Geometry check sheet. Reference: the model listing, model coordinates, mm. Face numbers are marked on the shaded views. A direction names the side the tool comes from. Give positions to 0.01 mm unless a question says otherwise; leave off trailing zeros. Order: outer loops, then holes, each group sorted by start corner. A loop starts at its lowest first (then second) coordinate and runs counter-clockwise, first axis right, second up. Notation, with made-up numbers: M 61,79 L 114,79 A29 cw 114,103 Z; hole C 24.25,65 d4. An arc over 180 degrees is marked long. Answer as CSV lines item,"result". Start each with the question number.
Q1. Section check A-A, the plane x = 60.4. Record the boundary of the cut face in (y, z).
Q2. Thickness scan on line 1 (Z direction, x = 37, y = 13.6); line 2 (Z direction, x = 20.5, y = 13.35); line 3 (X direction, y = 13.5, z = -188). Record the ranges inside material, lowest first.
Q3. Section check D-D, the plane z = -173. Record the boundary of the cut face in (x, y).
Q4. Go/stop test with flat-tipped pins: pin 1 (0.8 mm diameter, centred on y = 14, z = -108.5, fed in from +X); pin 2 (22 mm diameter, centred on x = 62, z = -86, fed in from -Y); pin 3 (1.3 mm diameter, centred on y = 14, z = -50.5, fed in from +X). Record where each tip stops, or that it passes through.
Q5. Set-up check for the marked faces 1 and 2: record each of +Z, -Z, +X, -X, +Y, -Y from which the full face is reachable in a straight line by a thin tool's end or side.
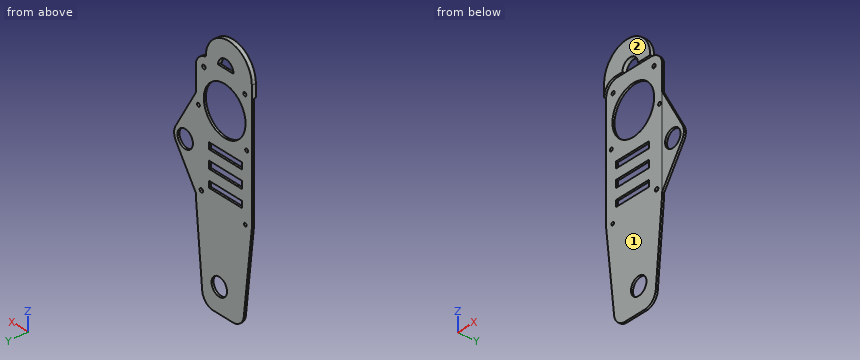
```python
from build123d import *

# Parameters (mm, degrees)
SKETCH1_R           = 2.875
SKETCH1_R_2         = 7
BOSS_EXTRUDE1_DEPTH = 24.5875
SKETCH4_W           = 66.272407177
SKETCH4_H           = 27.800260981
CUT_EXTRUDE2_DEPTH  = 20
FILLET3_R           = 10
FILLET4_R           = 10
BOSS_EXTRUDE3_START = -1.5875
BOSS_EXTRUDE3_DEPTH = 1.5875
SKETCH7_R           = 7
CUT_EXTRUDE3_DEPTH  = 1.5875
CUT_EXTRUDE4_START  = -10
SKETCH8_R           = 3
SKETCH8_R_2         = 18.9
SKETCH8_R_3         = 2.875
SKETCH8_R_4         = 7
CUT_EXTRUDE4_DEPTH  = 10
SKETCH9_W           = 229.1070397
SKETCH9_H           = 361.266964835
SKETCH9_R           = 1.388229101
SKETCH9_R_2         = 1.483383261
SKETCH9_R_3         = 1.314910669
SKETCH9_R_4         = 1.248623853
SKETCH9_R_5         = 1.255629307
SKETCH9_R_6         = 1.53911217
CUT_EXTRUDE5_DEPTH  = 13
SKETCH10_W          = 29.988446547
SKETCH10_H          = 5
SKETCH10_H_2        = 5.75
CUT_EXTRUDE6_DEPTH  = 22
SKETCH11_R          = 5.236653548
CUT_EXTRUDE7_DEPTH  = 10
BOSS_EXTRUDE4_START = -1.59
BOSS_EXTRUDE4_DEPTH = 1.59
SKETCH13_R          = 7
CUT_EXTRUDE8_DEPTH  = 41
SKETCH14_W          = 61.491848917
SKETCH14_H          = 35.587491391
CUT_EXTRUDE9_DEPTH  = 20
FILLET5_R           = 10
SKETCH16_W          = 163.723031551
SKETCH16_H          = 22.872070304
CUT_EXTRUDE11_DEPTH = 35
FILLET6_R           = 10
SKETCH17_R          = 1.53911217
SKETCH17_R_2        = 1.255629307
SKETCH17_R_3        = 1.3
SKETCH17_R_4        = 1.314910669
SKETCH17_R_5        = 1.388229101
SKETCH17_R_6        = 1.5
CUT_EXTRUDE12_DEPTH = 42
CUT_EXTRUDE13_START = -30
SKETCH18_R          = 18.9
CUT_EXTRUDE13_DEPTH = 30
BOSS_EXTRUDE5_DEPTH = 3.175


with BuildPart() as part:
    # Sketch1 → Boss-Extrude1 (new body)
    with BuildSketch(Plane(origin=(0, 0, 0), x_dir=(1, 0, 0), z_dir=(0, 1, 0))):
        with BuildLine():
            Line((42.32729629, 228.6), (10.454309325, 228.6))
            Line((10.454309325, 228.6), (0, 135.362739137))
            Line((0, 135.362739137), (0, 0))
            Line((0, 0), (24.327009544, 0))
            Line((24.327009544, 0), (50.8, 0))
            Line((50.8, 0), (50.8, 64.87909603))
            Line((50.8, 64.87909603), (50.8, 87.423477361))
            Line((50.8, 87.423477361), (50.8, 98.200996728))
            ThreePointArc((50.8, 98.200996728), (50.4, 101.000996728), (50.8, 103.800996728))
            Line((50.8, 103.800996728), (50.8, 104.488200565))
            Line((50.8, 104.488200565), (50.8, 120.619222808))
            Line((50.8, 120.619222808), (50.8, 135.362739137))
            Line((50.8, 135.362739137), (42.32729629, 228.6))
        make_face()
        with Locations(Location((24.101759227, 108.78493524, 0), (0, 0, 270))):
            Circle(SKETCH1_R, mode=Mode.SUBTRACT)
        with Locations(Location((29.504213454, 189.557234372, 0), (0, 0, 270))):
            Circle(SKETCH1_R_2, mode=Mode.SUBTRACT)
    extrude(amount=BOSS_EXTRUDE1_DEPTH)

    # Sketch4 → Cut-Extrude2 (cut)
    with BuildSketch(Plane(origin=(0, 0, -228.6), x_dir=(-1, 0, 0), z_dir=(0, 0, -1))):
        with Locations((-28.174690156, -1.980940155)):
            Rectangle(SKETCH4_W, SKETCH4_H)
    extrude(amount=-CUT_EXTRUDE2_DEPTH, mode=Mode.SUBTRACT)

    # Fillet3
    fillet3_edges = [part.edges().sort_by_distance(p)[0] for p in [
        (44.144746445, 5.959595168, -208.6),
    ]]
    fillet(fillet3_edges, radius=FILLET3_R)

    # Fillet4
    fillet4_edges = [part.edges().sort_by_distance(p)[0] for p in [
        (50.8, 12.29375, 0),
        (0, 12.29375, 0),
        (8.211791854, 5.959595168, -208.6),
    ]]
    fillet(fillet4_edges, radius=FILLET4_R)

    # Sketch6 → Boss-Extrude3 (add)
    with BuildSketch(Plane(origin=(0, 24.5875, 0), x_dir=(1, 0, 0), z_dir=(0, 1, 0)).offset(BOSS_EXTRUDE3_START)):
        with BuildLine():
            Line((50.8, 135.362739137), (50.8, 103.800996728))
            ThreePointArc((50.8, 103.800996728), (50.4, 101.000996728), (50.8, 98.200996728))
            Line((50.8, 98.200996728), (50.8, 61.124243317))
            Line((50.8, 61.124243317), (69.258211507, 96.360728536))
            ThreePointArc((69.258211507, 96.360728536), (70.393157133, 101.370875786), (68.890940865, 106.283413148))
            Line((68.890940865, 106.283413148), (50.8, 135.362739137))
        make_face()
    extrude(amount=BOSS_EXTRUDE3_DEPTH)

    # Sketch7 → Cut-Extrude3 (cut)
    with BuildSketch(Plane(origin=(0, 24.5875, 0), x_dir=(1, 0, 0), z_dir=(0, 1, 0))):
        with Locations(Location((60.4, 101.000996728, 0), (0, 0, 270))):
            Circle(SKETCH7_R)
    extrude(amount=-CUT_EXTRUDE3_DEPTH, mode=Mode.SUBTRACT)

    # Sketch8 → Cut-Extrude4 (cut)
    with BuildSketch(Plane(origin=(0, 24.5875, 0), x_dir=(1, 0, 0), z_dir=(0, 1, 0)).offset(CUT_EXTRUDE4_START)):
        with BuildLine():
            Line((10.454309325, 228.6), (0, 135.362739137))
            Line((0, 135.362739137), (0, 10))
            ThreePointArc((0, 10), (2.928932188, 2.928932188), (10, 0))
            Line((10, 0), (40.8, 0))
            ThreePointArc((40.8, 0), (47.871067812, 2.928932188), (50.8, 10))
            Line((50.8, 10), (50.8, 61.124243317))
            Line((50.8, 61.124243317), (69.258211507, 96.360728536))
            ThreePointArc((69.258211507, 96.360728536), (70.393157133, 101.370875786), (68.890940865, 106.283413148))
            Line((68.890940865, 106.283413148), (50.8, 135.362739137))
            Line((50.8, 135.362739137), (42.32729629, 228.6))
            Line((42.32729629, 228.6), (10.454309325, 228.6))
        make_face()
        with Locations(Location((9.492033273, 118.909935242, 0), (0, 0, 270))):
            Circle(SKETCH8_R, mode=Mode.SUBTRACT)
        with Locations(Location((24.583834565, 64.593886665, 0), (0, 0, 270))):
            Circle(SKETCH8_R_2, mode=Mode.SUBTRACT)
        with Locations(Location((24.101759227, 108.78493524, 0), (0, 0, 270))):
            Circle(SKETCH8_R_3, mode=Mode.SUBTRACT)
        with Locations((60.4, 101.000996728)):
            Circle(SKETCH8_R_4, mode=Mode.SUBTRACT)
        with Locations(Location((29.504213454, 189.557234372, 0), (0, 0, 270))):
            Circle(SKETCH8_R_4, mode=Mode.SUBTRACT)
    extrude(amount=CUT_EXTRUDE4_DEPTH, mode=Mode.SUBTRACT)

    # Sketch9 → Cut-Extrude5 (cut)
    with BuildSketch(Plane.XZ):
        with Locations((19.903204009, -125.752229467)):
            Rectangle(SKETCH9_W, SKETCH9_H)
        with Locations(Location((6.335590122, -44.288799513, 0), (0, 0, 270))):
            Circle(SKETCH9_R, mode=Mode.SUBTRACT)
        with Locations(Location((43.447673368, -42.868436544, 0), (0, 0, 270))):
            Circle(SKETCH9_R_2, mode=Mode.SUBTRACT)
        with Locations(Location((4.659546827, -82.793173401, 0), (0, 0, 270))):
            Circle(SKETCH9_R_3, mode=Mode.SUBTRACT)
        with Locations(Location((48.400988852, -71.551011715, 0), (0, 0, 270))):
            Circle(SKETCH9_R_4, mode=Mode.SUBTRACT)
        with Locations(Location((5.88467603, -135.103145298, 0), (0, 0, 270))):
            Circle(SKETCH9_R_5, mode=Mode.SUBTRACT)
        with Locations(Location((45.747747887, -129.863467374, 0), (0, 0, 270))):
            Circle(SKETCH9_R_6, mode=Mode.SUBTRACT)
    extrude(amount=-CUT_EXTRUDE5_DEPTH, mode=Mode.SUBTRACT)

    # Sketch10 → Cut-Extrude6 (cut)
    with BuildSketch(Plane(origin=(0, 24.5875, 0), x_dir=(1, 0, 0), z_dir=(0, 1, 0))):
        with Locations((23.779803557, 122.41493524)):
            Rectangle(SKETCH10_W, SKETCH10_H)
        with Locations((23.779803557, 108.78493524)):
            Rectangle(SKETCH10_W, SKETCH10_H_2)
        with Locations((23.779803557, 95.528937895)):
            Rectangle(SKETCH10_W, SKETCH10_H)
    extrude(amount=-CUT_EXTRUDE6_DEPTH, mode=Mode.SUBTRACT)

    # Sketch11 → Cut-Extrude7 (cut)
    with BuildSketch(Plane(origin=(0, 24.5875, 0), x_dir=(1, 0, 0), z_dir=(0, 1, 0))):
        with Locations((8.535526315, 118.29502971)):
            Circle(SKETCH11_R)
    extrude(amount=-CUT_EXTRUDE7_DEPTH, mode=Mode.SUBTRACT)

    # Sketch12 → Boss-Extrude4 (add)
    with BuildSketch(Plane(origin=(0, 14.5875, 0), x_dir=(1, 0, 0), z_dir=(0, 1, 0)).offset(BOSS_EXTRUDE4_START)):
        with BuildLine():
            Line((68.287536191, 107.148091395), (50.8, 133.900488173))
            Line((50.8, 133.900488173), (50.8, 103.800996728))
            ThreePointArc((50.8, 103.800996728), (58.520134646, 110.822712782), (68.287536191, 107.148091395))
        make_face()
        with BuildLine():
            Line((69.19540964, 105.759228466), (68.287536191, 107.148091395))
            ThreePointArc((68.287536191, 107.148091395), (58.520134646, 110.822712782), (50.8, 103.800996728))
            ThreePointArc((50.8, 103.800996728), (50.4, 101.000996728), (50.8, 98.200996728))
            ThreePointArc((50.8, 98.200996728), (59.211240578, 91.07190558), (69.067690563, 96.013899345))
            ThreePointArc((69.067690563, 96.013899345), (70.061182785, 98.419999404), (70.4, 101.000996728))
            ThreePointArc((70.4, 101.000996728), (70.094175994, 103.455167016), (69.19540964, 105.759228466))
        make_face()
        with BuildLine():
            ThreePointArc((69.067690563, 96.013899345), (59.211240578, 91.07190558), (50.8, 98.200996728))
            Line((50.8, 98.200996728), (50.8, 64.264230765))
            Line((50.8, 64.264230765), (69.067690563, 96.013899345))
        make_face()
    extrude(amount=BOSS_EXTRUDE4_DEPTH)

    # Sketch13 → Cut-Extrude8 (cut)
    with BuildSketch(Plane(origin=(0, 14.5875, 0), x_dir=(1, 0, 0), z_dir=(0, 1, 0))):
        with Locations(Location((60.4, 101.000996728, 0), (0, 0, 270))):
            Circle(SKETCH13_R)
    extrude(amount=-CUT_EXTRUDE8_DEPTH, mode=Mode.SUBTRACT)

    # Sketch14 → Cut-Extrude9 (cut)
    with BuildSketch(Plane(origin=(0, 0, -228.6), x_dir=(-1, 0, 0), z_dir=(0, 0, -1))):
        with Locations((-33.296946078, 21.381494753)):
            Rectangle(SKETCH14_W, SKETCH14_H)
    extrude(amount=-CUT_EXTRUDE9_DEPTH, mode=Mode.SUBTRACT)

    # Fillet5
    fillet5_edges = [part.edges().sort_by_distance(p)[0] for p in [
        (44.144746445, 13.79375, -208.6),
        (8.211791854, 13.79375, -208.6),
    ]]
    fillet(fillet5_edges, radius=FILLET5_R)

    # Sketch16 → Cut-Extrude11 (cut)
    with BuildSketch(Plane.XY):
        with Locations((6.935844153, 9.456999915)):
            Rectangle(SKETCH16_W, SKETCH16_H)
    extrude(amount=-CUT_EXTRUDE11_DEPTH, mode=Mode.SUBTRACT)

    # Fillet6
    fillet6_edges = [part.edges().sort_by_distance(p)[0] for p in [
        (0, 13.79375, -35),
        (50.8, 13.79375, -35),
    ]]
    fillet(fillet6_edges, radius=FILLET6_R)

    # Sketch17 → Cut-Extrude12 (cut)
    with BuildSketch(Plane.XZ):
        with Locations(Location((45.747747887, -129.863467374, 0), (0, 0, 270))):
            Circle(SKETCH17_R)
        with Locations(Location((5.88467603, -135.103145298, 0), (0, 0, 270))):
            Circle(SKETCH17_R_2)
        with Locations(Location((48.400988852, -71.551011715, 0), (0, 0, 270))):
            Circle(SKETCH17_R_3)
        with Locations(Location((4.659546827, -82.793173401, 0), (0, 0, 270))):
            Circle(SKETCH17_R_4)
        with Locations(Location((6.335590122, -44.288799513, 0), (0, 0, 270))):
            Circle(SKETCH17_R_5)
        with Locations(Location((43.447673368, -42.868436544, 0), (0, 0, 270))):
            Circle(SKETCH17_R_6)
    extrude(amount=-CUT_EXTRUDE12_DEPTH, mode=Mode.SUBTRACT)

    # Sketch18 → Cut-Extrude13 (cut)
    with BuildSketch(Plane(origin=(0, 24.5875, 0), x_dir=(1, 0, 0), z_dir=(0, 1, 0)).offset(CUT_EXTRUDE13_START)):
        with Locations(Location((24.583834565, 64.593886665, 0), (0, 0, 270))):
            Circle(SKETCH18_R)
    extrude(amount=CUT_EXTRUDE13_DEPTH, mode=Mode.SUBTRACT)

    # Sketch19 → Boss-Extrude5 (add)
    with BuildSketch(Plane(origin=(0, 14.5875, 0), x_dir=(1, 0, 0), z_dir=(0, 1, 0))):
        with BuildLine():
            ThreePointArc((10, 35), (2.928932188, 37.928932188), (0, 45))
            Line((0, 45), (0, 35))
            ThreePointArc((0, 35), (20.920362417, 14.10428472), (41.791401522, 35.049265202))
            ThreePointArc((41.791401522, 35.049265202), (41.296312411, 35.012323894), (40.8, 35))
            Line((40.8, 35), (30.546186564, 35))
            ThreePointArc((30.546186564, 35), (23.546186564, 28), (16.546186564, 35))
            Line((16.546186564, 35), (10, 35))
        make_face()
    extrude(amount=-BOSS_EXTRUDE5_DEPTH)


solid = part.part
```
Answer block:
1,outline,"M 13,-119.21 L 14.59,-119.21 L 14.59,-108 L 13,-108 Z; M 13,-94 L 14.59,-94 L 14.59,-80.95 L 13,-80.95 Z"
2,line 1,"z = -208.4 to -124.91, -119.91 to -111.66, -105.91 to -98.03, -93.03 to -78.84, -50.34 to -21.69"
2,line 2,"z = -208.6 to -124.91, -119.91 to -111.66, -105.91 to -98.03, -93.03 to -83.05, -46.14 to -35, -28.7 to -14.11"
2,line 3,"x = 5.9 to 22.68, 36.33 to 46.02"
3,outline,"M 4.22,13 L 47.38,13 L 47.38,14.59 L 4.22,14.59 Z"
4,pin 1,"stops at x = 67.67"
4,pin 2,"stops at y = 13"
4,pin 3,"stops at x = 50.8"
5,face 1,"-Z, +X, -Y"
5,face 2,"+Z, -Z, +X, -X, -Y"
